from build123d import *

# Parameters (mm, degrees)
BOSS_EXTRUDE1_DEPTH = 24.5
CUT_EXTRUDE1_DEPTH  = 26.12
LPATTERN1_DEPTH     = 24.5


# Read off the part's stored shape, not the designer's step: LPattern1
with BuildPart() as part:
    # Sketch1 → Boss-Extrude1 (new body)
    with BuildSketch(Plane.XY):
        Polygon((28.000000003, 7), (-39.373173928, 7), (-39.373173928, -0.249149017), (0.939234275, -0.249149017), (57.333339072, -0.249149017), (57.333339072, 7), align=None)
    extrude(amount=BOSS_EXTRUDE1_DEPTH)

    # Sketch2 → Cut-Extrude1 (cut)
    with BuildSketch(Plane.XY):
        with BuildLine():
            ThreePointArc((-6.881285782, 3.348371163), (-7.417069895, 3.826658598), (-7.671285782, 4.498371163))
            ThreePointArc((-7.671285782, 4.498371163), (-7.912320341, 6.04482582), (-8.981285782, 7.188037328))
            ThreePointArc((-8.981285782, 7.188037328), (-6.881285782, 7.762283268), (-4.781285782, 7.188037328))
            ThreePointArc((-4.781285782, 7.188037328), (-5.850251222, 6.04482582), (-6.091285782, 4.498371163))
            ThreePointArc((-6.091285782, 4.498371163), (-6.345501668, 3.826658598), (-6.881285782, 3.348371163))
        make_face()
    extrude(amount=CUT_EXTRUDE1_DEPTH, mode=Mode.SUBTRACT)

    # LPattern1 outline → LPattern1 (cut)
    with BuildSketch(Plane.XY):
        with BuildLine():
            ThreePointArc((-2.381285782, 3.348371163), (-1.845501668, 3.826658598), (-1.591285782, 4.498371163))
            ThreePointArc((-1.591285782, 4.498371163), (-1.419955599, 5.889231843), (-0.5655309, 7))
            Line((-0.5655309, 7), (-4.197040663, 7))
            ThreePointArc((-4.197040663, 7), (-3.342615965, 5.889231843), (-3.171285782, 4.498371163))
            ThreePointArc((-3.171285782, 4.498371163), (-2.917069895, 3.826658598), (-2.381285782, 3.348371163))
        make_face()
        with BuildLine():
            Line((53.4344691, 7), (49.802959337, 7))
            ThreePointArc((49.802959337, 7), (50.657384035, 5.889231843), (50.828714218, 4.498371163))
            ThreePointArc((50.828714218, 4.498371163), (51.082930105, 3.826658598), (51.618714218, 3.348371163))
            ThreePointArc((51.618714218, 3.348371163), (52.154498332, 3.826658598), (52.408714218, 4.498371163))
            ThreePointArc((52.408714218, 4.498371163), (52.580044401, 5.889231843), (53.4344691, 7))
        make_face()
        with BuildLine():
            Line((48.9344691, 7), (45.302959337, 7))
            ThreePointArc((45.302959337, 7), (46.157384035, 5.889231843), (46.328714218, 4.498371163))
            ThreePointArc((46.328714218, 4.498371163), (46.582930105, 3.826658598), (47.118714218, 3.348371163))
            ThreePointArc((47.118714218, 3.348371163), (47.654498332, 3.826658598), (47.908714218, 4.498371163))
            ThreePointArc((47.908714218, 4.498371163), (48.080044401, 5.889231843), (48.9344691, 7))
        make_face()
        with BuildLine():
            Line((44.4344691, 7), (40.802959337, 7))
            ThreePointArc((40.802959337, 7), (41.657384035, 5.889231843), (41.828714218, 4.498371163))
            ThreePointArc((41.828714218, 4.498371163), (42.082930105, 3.826658598), (42.618714218, 3.348371163))
            ThreePointArc((42.618714218, 3.348371163), (43.154498332, 3.826658598), (43.408714218, 4.498371163))
            ThreePointArc((43.408714218, 4.498371163), (43.580044401, 5.889231843), (44.4344691, 7))
        make_face()
        with BuildLine():
            Line((39.9344691, 7), (36.302959337, 7))
            ThreePointArc((36.302959337, 7), (37.157384035, 5.889231843), (37.328714218, 4.498371163))
            ThreePointArc((37.328714218, 4.498371163), (37.582930105, 3.826658598), (38.118714218, 3.348371163))
            ThreePointArc((38.118714218, 3.348371163), (38.654498332, 3.826658598), (38.908714218, 4.498371163))
            ThreePointArc((38.908714218, 4.498371163), (39.080044401, 5.889231843), (39.9344691, 7))
        make_face()
        with BuildLine():
            Line((35.4344691, 7), (31.802959337, 7))
            ThreePointArc((31.802959337, 7), (32.657384035, 5.889231843), (32.828714218, 4.498371163))
            ThreePointArc((32.828714218, 4.498371163), (33.082930105, 3.826658598), (33.618714218, 3.348371163))
            ThreePointArc((33.618714218, 3.348371163), (34.154498332, 3.826658598), (34.408714218, 4.498371163))
            ThreePointArc((34.408714218, 4.498371163), (34.580044401, 5.889231843), (35.4344691, 7))
        make_face()
        with BuildLine():
            Line((30.9344691, 7), (27.302959337, 7))
            ThreePointArc((27.302959337, 7), (28.157384035, 5.889231843), (28.328714218, 4.498371163))
            ThreePointArc((28.328714218, 4.498371163), (28.582930105, 3.826658598), (29.118714218, 3.348371163))
            ThreePointArc((29.118714218, 3.348371163), (29.654498332, 3.826658598), (29.908714218, 4.498371163))
            ThreePointArc((29.908714218, 4.498371163), (30.080044401, 5.889231843), (30.9344691, 7))
        make_face()
        with BuildLine():
            Line((26.4344691, 7), (22.802959337, 7))
            ThreePointArc((22.802959337, 7), (23.657384035, 5.889231843), (23.828714218, 4.498371163))
            ThreePointArc((23.828714218, 4.498371163), (24.082930105, 3.826658598), (24.618714218, 3.348371163))
            ThreePointArc((24.618714218, 3.348371163), (25.154498332, 3.826658598), (25.408714218, 4.498371163))
            ThreePointArc((25.408714218, 4.498371163), (25.580044401, 5.889231843), (26.4344691, 7))
        make_face()
        with BuildLine():
            Line((21.9344691, 7), (18.302959337, 7))
            ThreePointArc((18.302959337, 7), (19.157384035, 5.889231843), (19.328714218, 4.498371163))
            ThreePointArc((19.328714218, 4.498371163), (19.582930105, 3.826658598), (20.118714218, 3.348371163))
            ThreePointArc((20.118714218, 3.348371163), (20.654498332, 3.826658598), (20.908714218, 4.498371163))
            ThreePointArc((20.908714218, 4.498371163), (21.080044401, 5.889231843), (21.9344691, 7))
        make_face()
        with BuildLine():
            Line((17.4344691, 7), (13.802959337, 7))
            ThreePointArc((13.802959337, 7), (14.657384035, 5.889231843), (14.828714218, 4.498371163))
            ThreePointArc((14.828714218, 4.498371163), (15.082930105, 3.826658598), (15.618714218, 3.348371163))
            ThreePointArc((15.618714218, 3.348371163), (16.154498332, 3.826658598), (16.408714218, 4.498371163))
            ThreePointArc((16.408714218, 4.498371163), (16.580044401, 5.889231843), (17.4344691, 7))
        make_face()
        with BuildLine():
            Line((12.9344691, 7), (9.302959337, 7))
            ThreePointArc((9.302959337, 7), (10.157384035, 5.889231843), (10.328714218, 4.498371163))
            ThreePointArc((10.328714218, 4.498371163), (10.582930105, 3.826658598), (11.118714218, 3.348371163))
            ThreePointArc((11.118714218, 3.348371163), (11.654498332, 3.826658598), (11.908714218, 4.498371163))
            ThreePointArc((11.908714218, 4.498371163), (12.080044401, 5.889231843), (12.9344691, 7))
        make_face()
        with BuildLine():
            Line((8.4344691, 7), (4.802959337, 7))
            ThreePointArc((4.802959337, 7), (5.657384035, 5.889231843), (5.828714218, 4.498371163))
            ThreePointArc((5.828714218, 4.498371163), (6.082930105, 3.826658598), (6.618714218, 3.348371163))
            ThreePointArc((6.618714218, 3.348371163), (7.154498332, 3.826658598), (7.408714218, 4.498371163))
            ThreePointArc((7.408714218, 4.498371163), (7.580044401, 5.889231843), (8.4344691, 7))
        make_face()
        with BuildLine():
            Line((3.9344691, 7), (0.302959337, 7))
            ThreePointArc((0.302959337, 7), (1.157384035, 5.889231843), (1.328714218, 4.498371163))
            ThreePointArc((1.328714218, 4.498371163), (1.582930105, 3.826658598), (2.118714218, 3.348371163))
            ThreePointArc((2.118714218, 3.348371163), (2.654498332, 3.826658598), (2.908714218, 4.498371163))
            ThreePointArc((2.908714218, 4.498371163), (3.080044401, 5.889231843), (3.9344691, 7))
        make_face()
        with BuildLine():
            ThreePointArc((-26.881285782, 3.348371163), (-26.345501668, 3.826658598), (-26.091285782, 4.498371163))
            ThreePointArc((-26.091285782, 4.498371163), (-25.919955599, 5.889231843), (-25.0655309, 7))
            Line((-25.0655309, 7), (-28.697040663, 7))
            ThreePointArc((-28.697040663, 7), (-27.842615965, 5.889231843), (-27.671285782, 4.498371163))
            ThreePointArc((-27.671285782, 4.498371163), (-27.417069895, 3.826658598), (-26.881285782, 3.348371163))
        make_face()
        with BuildLine():
            ThreePointArc((-36.091285782, 4.498371163), (-35.919955599, 5.889231843), (-35.0655309, 7))
            Line((-35.0655309, 7), (-38.697040663, 7))
            ThreePointArc((-38.697040663, 7), (-37.842615965, 5.889231843), (-37.671285782, 4.498371163))
            ThreePointArc((-37.671285782, 4.498371163), (-37.417069895, 3.826658598), (-36.881285782, 3.348371163))
            ThreePointArc((-36.881285782, 3.348371163), (-36.345501668, 3.826658598), (-36.091285782, 4.498371163))
        make_face()
        with BuildLine():
            ThreePointArc((-31.091285782, 4.498371163), (-30.919955599, 5.889231843), (-30.0655309, 7))
            Line((-30.0655309, 7), (-33.697040663, 7))
            ThreePointArc((-33.697040663, 7), (-32.842615965, 5.889231843), (-32.671285782, 4.498371163))
            ThreePointArc((-32.671285782, 4.498371163), (-32.417069895, 3.826658598), (-31.881285782, 3.348371163))
            ThreePointArc((-31.881285782, 3.348371163), (-31.345501668, 3.826658598), (-31.091285782, 4.498371163))
        make_face()
        with BuildLine():
            Line((-10.0655309, 7), (-13.697040663, 7))
            ThreePointArc((-13.697040663, 7), (-12.842615965, 5.889231843), (-12.671285782, 4.498371163))
            ThreePointArc((-12.671285782, 4.498371163), (-12.417069895, 3.826658598), (-11.881285782, 3.348371163))
            ThreePointArc((-11.881285782, 3.348371163), (-11.345501668, 3.826658598), (-11.091285782, 4.498371163))
            ThreePointArc((-11.091285782, 4.498371163), (-10.919955599, 5.889231843), (-10.0655309, 7))
        make_face()
        with BuildLine():
            Line((-15.0655309, 7), (-18.697040663, 7))
            ThreePointArc((-18.697040663, 7), (-17.842615965, 5.889231843), (-17.671285782, 4.498371163))
            ThreePointArc((-17.671285782, 4.498371163), (-17.417069895, 3.826658598), (-16.881285782, 3.348371163))
            ThreePointArc((-16.881285782, 3.348371163), (-16.345501668, 3.826658598), (-16.091285782, 4.498371163))
            ThreePointArc((-16.091285782, 4.498371163), (-15.919955599, 5.889231843), (-15.0655309, 7))
        make_face()
        with BuildLine():
            Line((-20.0655309, 7), (-23.697040663, 7))
            ThreePointArc((-23.697040663, 7), (-22.842615965, 5.889231843), (-22.671285782, 4.498371163))
            ThreePointArc((-22.671285782, 4.498371163), (-22.417069895, 3.826658598), (-21.881285782, 3.348371163))
            ThreePointArc((-21.881285782, 3.348371163), (-21.345501668, 3.826658598), (-21.091285782, 4.498371163))
            ThreePointArc((-21.091285782, 4.498371163), (-20.919955599, 5.889231843), (-20.0655309, 7))
        make_face()
    extrude(amount=LPATTERN1_DEPTH, mode=Mode.SUBTRACT)


solid = part.part
Input: part model. Units: mm. Frame: model coordinates. Give positions to 0.01 mm unless a question says otherwise; leave off trailing zeros. Answer as a JSON object with one key per item and string values. Group by question number.
Q1. Mould query, pull axis X, two halves, no side actions, for faces 1 (the face through (8, 3, 24.5)), 2 (the face through (21.073, 5.871, 12.078)). Classes: pulls with the +X half, pulls with the -X half, needs draft (parallel to the pull), parting line crosses it, or undercut.
Q2. Cut plane A-A, the plane y = 5.75. Count the separate pieces of the cut face and the enclosed holes in it, then the cut area to 3 significant figures.
Q3. Line query: probe 1 along Y at (x, z) = (28, 15); probe 2 along Y at (x, z) = (-2, 9.5). Output: solid intervals per line, ascending.
Results:
{
 "1": {"face 1": "needs draft", "face 2": "undercut"},
 "2": {"separate pieces": "21", "enclosed holes": "0", "area": "1,480 mm^2"},
 "3": {"probe 1": "-0.25 to 6.21", "probe 2": "-0.25 to 3.64"}
}
